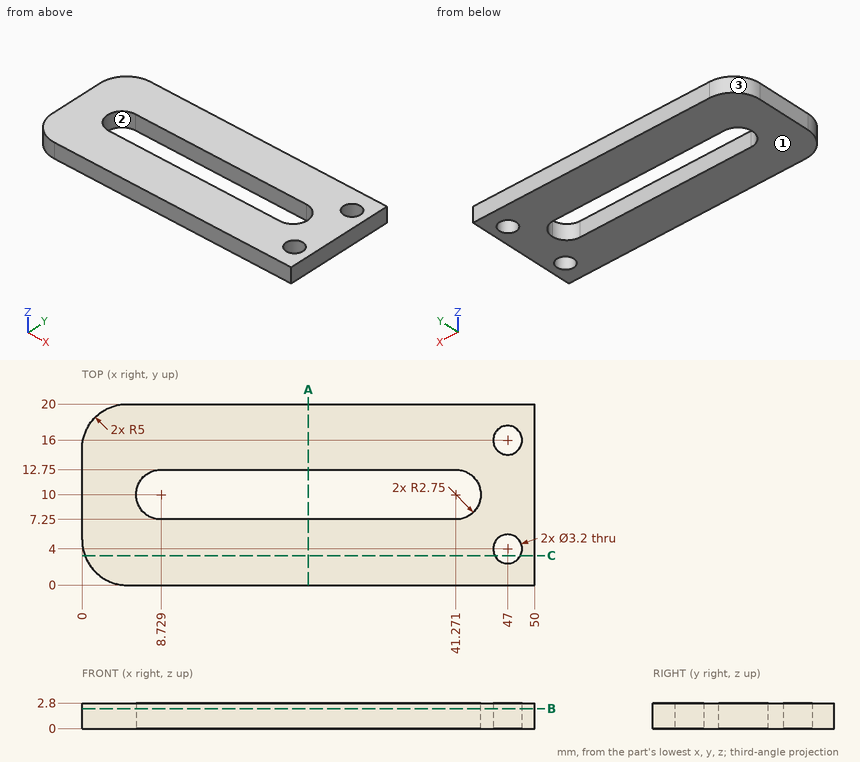
Geometry check sheet. Reference: drawing and pictorial views, mm from the part's lowest x, y, z. Give positions to 0.01 mm unless a question says otherwise; leave off trailing zeros. Order: outer loops, then holes, each group sorted by start corner. A loop starts at its lowest first (then second) coordinate and runs counter-clockwise, first axis right, second up.
1. Thickness scan on L1, parallel to Y at x = 47, z = 1.2; L2, parallel to Y at x = 21.5, z = 0.8; L3, parallel to X at y = 16.5, z = 1.9. Record the ranges inside material, lowest first.
2. Section check B-B, the plane z = 2.2. Enter the section's corners in (x, y).
3. Release check for a two-part mould opening along X. For the marked faces 1, 2 and 3 record: pulls with the +X half, pulls with the -X half, needs draft (parallel to the pull), parting line crosses it, or undercut.
4. Gauge pin test, flat end, axial feed: pin 1 Ø1.9 at (x, y) = (47, 4) entering from +Z. Record the tip position at first contact, or that the pin passes through.
5. Section check A-A, the plane x = 25. Enter the section's corners in (y, z), and give its area (3 significant figures).
6. Section check C-C, the plane y = 3.25. Enter the section's corners in (x, z).
Values follow:
1. L1: y = 0 to 2.4, 5.6 to 14.4, 17.6 to 20
1. L2: y = 0 to 7.25, 12.75 to 20
1. L3: x = 0.23 to 45.48, 48.52 to 50
2. outline: (0, 5) arc R5 ccw to (5, 0) - (50, 0) - (50, 20) - (5, 20) arc R5 ccw to (0, 15) - close; hole (8.73, 7.25) - (41.27, 7.25) arc R2.75 ccw to (44.02, 10) arc R2.75 ccw to (41.27, 12.75) - (8.73, 12.75) arc R2.75 ccw to start; hole circle Ø3.2 at (47, 4); hole circle Ø3.2 at (47, 16)
3. face 1: needs draft
3. face 2: undercut
3. face 3: pulls with the -X half
4. pin 1: passes through
5. outline: (0, 0) - (7.25, 0) - (7.25, 2.8) - (0, 2.8) - close; (12.75, 0) - (20, 0) - (20, 2.8) - (12.75, 2.8) - close
5. area: 40.6 mm2
6. outline: (0.32, 0) - (45.59, 0) - (45.59, 2.8) - (0.32, 2.8) - close; (48.41, 0) - (50, 0) - (50, 2.8) - (48.41, 2.8) - close
